from build123d import *

# Parameters (mm, degrees)
SKETCH1_R           = 16
SKETCH1_R_2         = 5
SKETCH1_R_3         = 1.975
BOSS_EXTRUDE1_DEPTH = 3.5
SKETCH2_R           = 16
BOSS_EXTRUDE2_DEPTH = 1
SKETCH3_R           = 16
SKETCH3_R_2         = 11.25
BOSS_EXTRUDE3_DEPTH = 6
SKETCH4_W           = 32
SKETCH4_H           = 1
CUT_EXTRUDE1_DEPTH  = 6
SKETCH5_R           = 7
CUT_EXTRUDE2_DEPTH  = 1


with BuildPart() as part:
    # Sketch1 → Boss-Extrude1 (new body)
    with BuildSketch(Plane(origin=(0, 0, 0), x_dir=(1, 0, 0), z_dir=(0, 1, 0))):
        with Locations(Location((0, 0, 0), (0, 0, 270))):
            Circle(SKETCH1_R)
        with Locations(Location((0, 0, 0), (0, 0, 270))):
            Circle(SKETCH1_R_2, mode=Mode.SUBTRACT)
        with Locations(Location((0, 12.5, 0), (0, 0, 270))):
            Circle(SKETCH1_R_3, mode=Mode.SUBTRACT)
        with Locations(Location((12.5, 0, 0), (0, 0, 270))):
            Circle(SKETCH1_R_3, mode=Mode.SUBTRACT)
        with Locations(Location((0, -12.5, 0), (0, 0, 270))):
            Circle(SKETCH1_R_3, mode=Mode.SUBTRACT)
        with Locations(Location((-12.5, 0, 0), (0, 0, 270))):
            Circle(SKETCH1_R_3, mode=Mode.SUBTRACT)
    extrude(amount=BOSS_EXTRUDE1_DEPTH)

    # Sketch2 → Boss-Extrude2 (add)
    with BuildSketch(Plane(origin=(0, 3.5, 0), x_dir=(1, 0, 0), z_dir=(0, 1, 0))):
        with Locations(Location((0, 0, 0), (0, 0, 270))):
            Circle(SKETCH2_R)
    extrude(amount=BOSS_EXTRUDE2_DEPTH)

    # Sketch3 → Boss-Extrude3 (add)
    with BuildSketch(Plane(origin=(0, 4.5, 0), x_dir=(1, 0, 0), z_dir=(0, 1, 0))):
        with Locations(Location((0, 0, 0), (0, 0, 270))):
            Circle(SKETCH3_R)
        with Locations(Location((0, 0, 0), (0, 0, 270))):
            Circle(SKETCH3_R_2, mode=Mode.SUBTRACT)
    extrude(amount=BOSS_EXTRUDE3_DEPTH)

    # Sketch4 → Cut-Extrude1 (cut)
    with BuildSketch(Plane(origin=(0, 10.5, 0), x_dir=(1, 0, 0), z_dir=(0, 1, 0))):
        Rectangle(SKETCH4_W, SKETCH4_H)
    extrude(amount=-CUT_EXTRUDE1_DEPTH, mode=Mode.SUBTRACT)

    # Sketch5 → Cut-Extrude2 (cut)
    with BuildSketch(Plane(origin=(0, 4.5, 0), x_dir=(1, 0, 0), z_dir=(0, 1, 0))):
        with Locations(Location((0, 0, 0), (0, 0, 270))):
            Circle(SKETCH5_R)
    extrude(amount=-CUT_EXTRUDE2_DEPTH, mode=Mode.SUBTRACT)


solid = part.part
Geometry check sheet. Reference: the model listing, model coordinates, mm. A direction names the side the tool comes from. Give positions to 0.01 mm unless a question says otherwise; leave off trailing zeros. Write each loop counter-clockwise with the first axis right and the second up, starting at its lowest first coordinate (ties: lowest second). Pieces come first, ordered by that corner, then holes. Notation, with made-up numbers: M 67.25,76 L 86.25,76 A24 ccw 86.25,103 Z; hole C -32,-33 d6. An arc over 180 degrees is marked long. Answer as CSV lines item,"result". Start each with the question number.
Q1. Section check B-B, the plane x = 0. Record the cut outline in (y, z) (3 decimals), then the cut area to 3 significant figures.
Q2. Section check D-D, the plane y = 2.5. Record the cut outline in (x, z) (3 decimals), then the cut area to 3 significant figures.
Q3. Material ranges on L1, parallel to X at y = 1.3, z = 0 (3 decimals); L2, parallel to X at y = 3.95, z = 0; L3, parallel to Y at x = 2, z = 9, recorded low to high.
Q4. Release check for a two-part mould opening along Z. For faces 1 (the face through (-15.62, 5.18, -3.47)), 2 (the face through (0, 10.5, -12)), 3 (the face through (14, 8, -0.5)) record: pulls with the +Z half, pulls with the -Z half, needs draft (parallel to the pull), parting line crosses it, or undercut.
Q5. Tool access check on faces 4 (the face through (-14, 8, -0.5)), 5 (the face through (0, 3.5, 12)), 6 (the face through (4, 0, -4)), 7 (the face through (0.24, 7.458, -11.247)), 8 (the face through (-4.88, 1.73, -1.08)). Record the directions out of +Z, -Z, +X, -X, +Y, -Y that give a thin tool (end or side, any length) a straight path to the whole face; none if there is none.
Q6. Section check C-C, the plane z = 3.5. Record the cut outline in (x, y), then the cut area to 3 significant figures.
Q7. Go/stop test with flat-tipped pins: pin 1 (1 mm diameter, centred on x = -2.5, y = 8, fed in from -Z); pin 2 (8 mm diameter, centred on x = 7, z = -1, fed in from +Y); pin 3 (7 mm diameter, centred on x = -2, z = 2.5, fed in from +Y). Record where each tip stops, or that it passes through.
Geometry says:
1,outline,"M 0,-16 L 10.5,-16 L 10.5,-11.25 L 4.5,-11.25 L 4.5,-7 L 3.5,-7 L 3.5,-5 L 0,-5 L 0,-10.525 L 3.5,-10.525 L 3.5,-14.475 L 0,-14.475 Z; M 0,5 L 3.5,5 L 3.5,7 L 4.5,7 L 4.5,11.25 L 10.5,11.25 L 10.5,16 L 0,16 L 0,14.475 L 3.5,14.475 L 3.5,10.525 L 0,10.525 Z"
1,area,"124 mm^2"
2,outline,"C 0,0 d32; hole C -12.5,0 d3.95; hole C 0,0 d10; hole C 0,-12.5 d3.95; hole C 0,12.5 d3.95; hole C 12.5,0 d3.95"
2,area,"677 mm^2"
3,L1,"-16 to -14.475, -10.525 to -5, 5 to 10.525, 14.475 to 16"
3,L2,"-16 to -7, 7 to 16"
3,L3,"0 to 4.5"
4,face 1,"parting line crosses it"
4,face 2,"needs draft"
4,face 3,"undercut"
5,face 4,"+X, -X, +Y"
5,face 5,"-Y"
5,face 6,"+Z, -Z, +X, -X, -Y"
5,face 7,"+Y"
5,face 8,"+Y, -Y"
6,outline,"M -15.61,0 L -3.57,0 L -3.57,3.5 L -6.06,3.5 L -6.06,4.5 L -10.69,4.5 L -10.69,10.5 L -15.61,10.5 Z; M 3.57,0 L 15.61,0 L 15.61,10.5 L 10.69,10.5 L 10.69,4.5 L 6.06,4.5 L 6.06,3.5 L 3.57,3.5 Z"
6,area,"162 mm^2"
7,pin 1,"z = -15.87"
7,pin 2,"y = 4.5"
7,pin 3,"y = 3.5"
